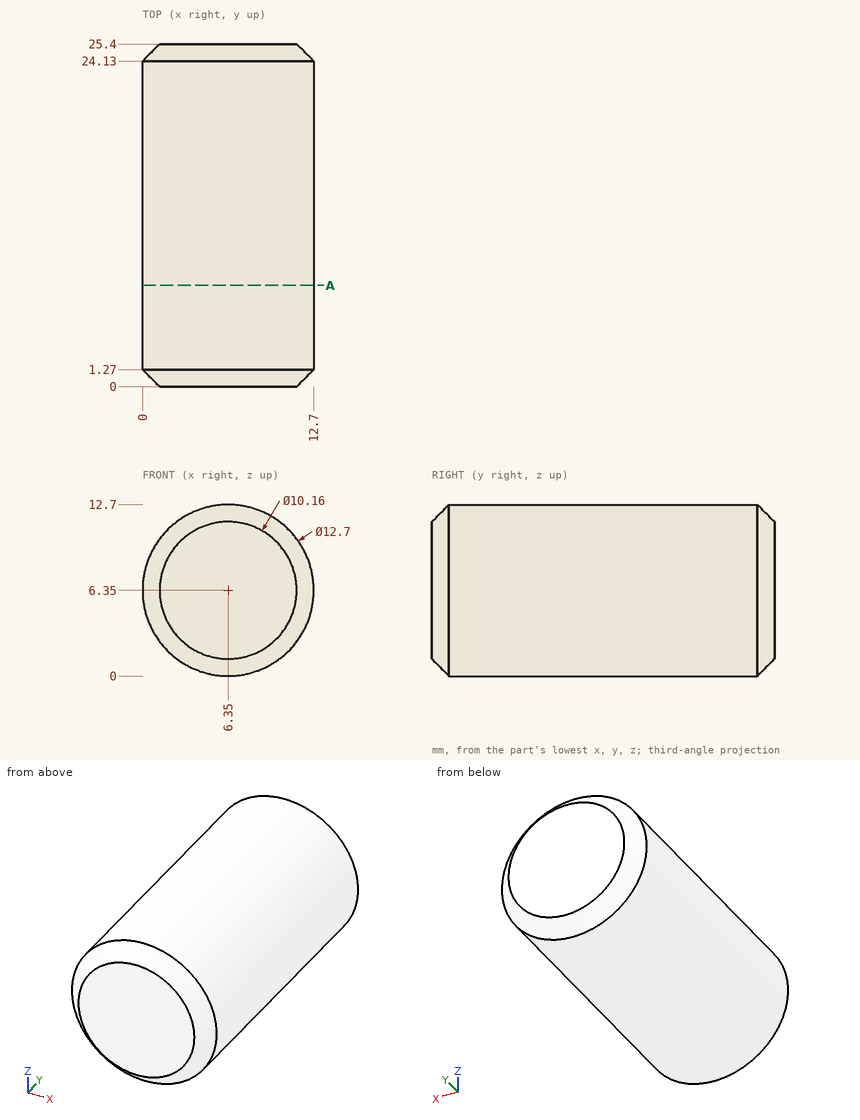
Geometry check sheet. Reference: drawing and pictorial views, mm from the part's lowest x, y, z. Give positions to 0.01 mm unless a question says otherwise; leave off trailing zeros. Write each loop counter-clockwise with the first axis right and the second up, starting at its lowest first coordinate (ties: lowest second). Pieces come first, ordered by that corner, then holes. Notation, with made-up numbers: (49, -14.75) -> (62, -14.75) arc R12 ccw to (62, 0.25) -> close; hole circle Ø4 at (73, 21). An arc over 180 degrees is marked (long way). One line per item, written item: value. Start each with the question number.
Item 1: Material ranges on probe 1 along Z at (x, y) = (6.5, 12.25); probe 2 along X at (y, z) = (22.75, 2.5); probe 3 along X at (y, z) = (6, 4), recorded low to high. Write a range as from..to.
Item 2: Gauge pin test, flat ends, axial feed: pin 1 (1.5 mm diameter, centred on y = 13, z = 2.5, fed in from +X); pin 2 (1.5 mm diameter, centred on y = 21.5, z = 7.5, fed in from -X); pin 3 (5 mm diameter, centred on x = 10, y = 13.5, fed in from +Z) (3 decimals). Record the tip position at first contact, or that the pin passes through.
Item 3: Section check A-A on y = 7.5. Record the cut outline in (x, z).
Results list:
1. probe 1: 0..12.7
1. probe 2: 1.3..11.4
1. probe 3: 0.45..12.25
2. pin 1: x = 11.89
2. pin 2: x = 0.01
2. pin 3: z = 12.595
3. outline: circle Ø12.7 at (6.35, 6.35)
